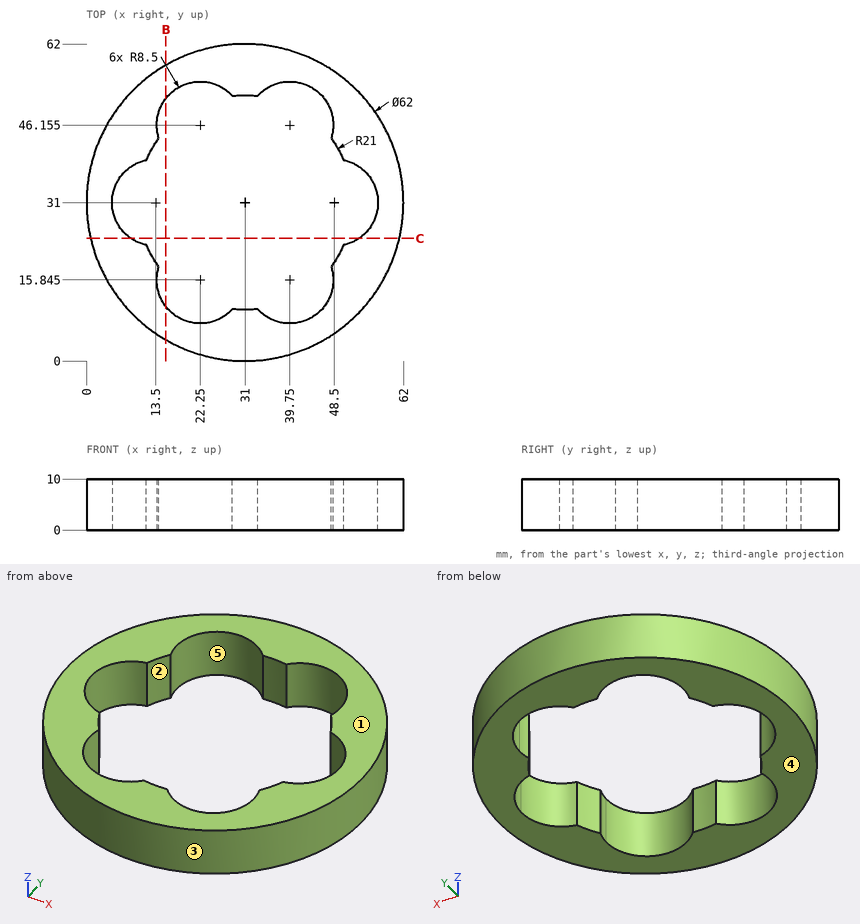
Design review of the part shown in the three views and the two pictorial views. Dimensions are in mm from the part's minimum x, y and z. A direction names the side the tool comes from. Round coordinates to 2 decimals unless told otherwise and drop trailing zeros. Write each loop counter-clockwise with the first axis right and the second up, starting at its lowest first coordinate (ties: lowest second). Pieces come first, ordered by that corner, then holes. Notation, with made-up numbers: M -27,32 L -19,32 A28 ccw -19,64 Z; hole C 47,22.25 d4. An arc over 180 degrees is marked long. One line per item, written item: value. Start each with the question number.
1. For the marked faces 1 and 2, list the 3-axis set-ups (+Z, -Z, +X, -X, +Y, -Y) from which the entire face can be reached by the end or side of a thin tool; tool diameter is ignored.
2. Clearance check with flat-ended pins moving along their axes: P1, Ø6, axis at y = 23, z = 5, coming from the -X side; P2, Ø6, axis at x = 53, z = 3, coming from the +Y side (1 decimal); P3, Ø6, axis at x = 38, z = 5, coming from the -Y side. State where each tip first meets the part, or that it passes through.
3. To check wall thickness, follow probe 1 along X at (y, z) = (54, 2) (1 decimal); probe 2 along X at (y, z) = (30.5, 1) (1 decimal); probe 3 along X at (y, z) = (16, 9). State the ranges of each line that lie inside material, in increasing order. Write a range as from..to.
4. Take a section at C-C on y = 24. State the section outline as (x, z) points.
5. Take a section at B-B on x = 15.5. State the section outline as (y, z) points.
6. Draft analysis for pull direction Y (two halves, no side actions). For the marked faces 3, 4 and 5, state which applies: pulls with the +Y half, pulls with the -Y half, needs draft (parallel to the pull), parting line crosses it, or undercut.
Computed:
1. face 1: +Z, +X, -X, +Y, -Y
1. face 2: +Z, -Z
2. P1: stops at x = 0.41
2. P2: stops at y = 55.5
2. P3: stops at y = 0.26
3. probe 1: x = 10.2..19, 25.5..36.5, 43..51.8
3. probe 2: x = 0..5, 57..62
3. probe 3: x = 3.87..13.75, 48.25..58.13
4. outline: M 0.8,0 L 8.68,0 L 8.68,10 L 0.8,10 Z; M 53.32,0 L 61.2,0 L 61.2,10 L 53.32,10 Z
5. outline: M 4.15,0 L 10.68,0 L 10.68,10 L 4.15,10 Z; M 51.32,0 L 57.85,0 L 57.85,10 L 51.32,10 Z
6. face 3: parting line crosses it
6. face 4: needs draft
6. face 5: undercut
